Work out the finished part from the listing and answer in its coordinate system (mm). Coordinates: 2 decimals unless noted, no trailing zeros. Order: outer loops, then holes, each group sorted by start corner. A loop starts at its lowest first (then second) coordinate and runs counter-clockwise, first axis right, second up. Notation, with made-up numbers: (18, -34.5) -> (74, -34.5) arc R24 ccw to (74, -20.5) -> close; hole circle Ø7 at (-13, 84). An arc over 180 degrees is marked (long way). Answer as CSV lines item,"result". Start each with the question number.
Item 1: Straight lines are drawn through the part: L1, parallel to Y at x = 740.5, z = 2.5 (3 decimals); L2, parallel to X at y = 1, z = 1.5; L3, parallel to X at y = -0.5, z = -1.5. For each, find the intervals that lie inside material, in ascending order.
Item 2: Section B-B (x = 104.5) is taken. Write down the section's boundary in (y, z) (3 decimals).
Item 3: Section A-A (y = 0) is taken. Write down the section's boundary in (x, z) (3 decimals).
Item 4: This flat-tipped pin is pushed along its axis until it touches: pin 1 Ø4 at (y, z) = (3.5, 0.5) entering from -X. Where does it stop, or does it pass through?
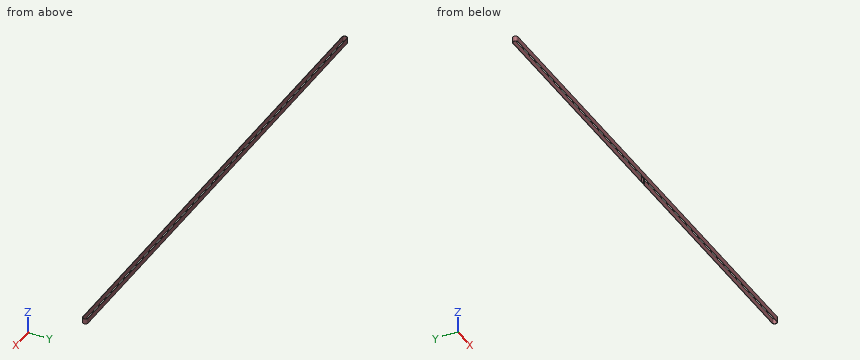
Autodesk Inventor part; units mm, degrees
ref_plane "YZ Plane" through (0, 0, 0) normal (1, 0, 0) x (0, 1, 0)
ref_plane "XZ Plane" through (0, 0, 0) normal (0, 1, 0) x (-1, 0, 0)
ref_plane "XY Plane" through (0, 0, 0) normal (0, 0, 1) x (1, 0, 0)
sketch "_____1" plane through (0, 0, 0) normal (0, 0, 1) x (1, 0, 0)
  arc A0 (0, 4.515) -> (0, -4.515) centre (0, 0) ccw
  line L0 (0, -4.515) -> (837, -4.515)
  arc A1 (837, -4.515) -> (837, 4.515) centre (837, 0) ccw
  line L1 (837, 4.515) -> (0, 4.515)
  arc A2 (0, 3.885) -> (0, -3.885) centre (0, 0) ccw
  line L2 (0, -3.885) -> (837, -3.885)
  arc A3 (837, -3.885) -> (837, 3.885) centre (837, 0) ccw
  line L3 (837, 3.885) -> (0, 3.885)
extrude "Extrusion1" add sketch "_____1" along normal mid plane 9
sketch "_____2" plane through (0, 0, 0) normal (0, 0, 1) x (1, 0, 0)
  line L0 (413.5, 4.515) -> (413.5, 3.885)
  line L1 (413.5, 3.885) -> (413.7598, 3.885)
  arc A0 (413.9085, 3.7546) -> (413.7598, 3.885) centre (413.7598, 3.735) ccw
  arc A1 (413.9085, 3.7546) -> (414.0011, 3.4468) centre (414.9, 3.885) ccw
  arc A2 (414.0011, 3.4468) -> (414.9989, 3.4468) centre (414.5, 3.69) ccw
  arc A3 (414.9989, 3.4468) -> (415.0915, 3.7546) centre (414.1, 3.885) ccw
  arc A4 (415.2402, 3.885) -> (415.0915, 3.7546) centre (415.2402, 3.735) ccw
  line L2 (415.2402, 3.885) -> (415.7598, 3.885)
  arc A5 (415.9085, 3.7546) -> (415.7598, 3.885) centre (415.7598, 3.735) ccw
  arc A6 (415.9085, 3.7546) -> (416.0011, 3.4468) centre (416.9, 3.885) ccw
  arc A7 (416.0011, 3.4468) -> (416.9989, 3.4468) centre (416.5, 3.69) ccw
  arc A8 (416.9989, 3.4468) -> (417.0915, 3.7546) centre (416.1, 3.885) ccw
  arc A9 (417.2402, 3.885) -> (417.0915, 3.7546) centre (417.2402, 3.735) ccw
  line L3 (417.2402, 3.885) -> (417.7598, 3.885)
  arc A10 (417.9085, 3.7546) -> (417.7598, 3.885) centre (417.7598, 3.735) ccw
  arc A11 (417.9085, 3.7546) -> (418.0011, 3.4468) centre (418.9, 3.885) ccw
  arc A12 (418.0011, 3.4468) -> (418.9989, 3.4468) centre (418.5, 3.69) ccw
  arc A13 (418.9989, 3.4468) -> (419.0915, 3.7546) centre (418.1, 3.885) ccw
  arc A14 (419.2402, 3.885) -> (419.0915, 3.7546) centre (419.2402, 3.735) ccw
  line L4 (419.2402, 3.885) -> (419.7598, 3.885)
  arc A15 (419.9085, 3.7546) -> (419.7598, 3.885) centre (419.7598, 3.735) ccw
  arc A16 (419.9085, 3.7546) -> (420.0011, 3.4468) centre (420.9, 3.885) ccw
  arc A17 (420.0011, 3.4468) -> (420.9989, 3.4468) centre (420.5, 3.69) ccw
  arc A18 (420.9989, 3.4468) -> (421.0915, 3.7546) centre (420.1, 3.885) ccw
  arc A19 (421.2402, 3.885) -> (421.0915, 3.7546) centre (421.2402, 3.735) ccw
  line L5 (421.2402, 3.885) -> (421.7598, 3.885)
  arc A20 (421.9085, 3.7546) -> (421.7598, 3.885) centre (421.7598, 3.735) ccw
  arc A21 (421.9085, 3.7546) -> (422.0011, 3.4468) centre (422.9, 3.885) ccw
  arc A22 (422.0011, 3.4468) -> (422.9989, 3.4468) centre (422.5, 3.69) ccw
  arc A23 (422.9989, 3.4468) -> (423.0915, 3.7546) centre (422.1, 3.885) ccw
  arc A24 (423.2402, 3.885) -> (423.0915, 3.7546) centre (423.2402, 3.735) ccw
  line L6 (423.2402, 3.885) -> (423.5, 3.885)
  line L7 (423.5, 3.885) -> (423.5, 4.515)
  line L8 (423.5, 4.515) -> (413.5, 4.515)
extrude "Extrusion2" add sketch "_____2" along normal mid plane 9
properties part number "GBN1700MR2-90_info-1-13-13"
Checked values:
1,L1,"y = -4.515 to -3.885, 3.885 to 4.515"
1,L2,"x = -4.4 to -3.75, 840.75 to 841.4"
1,L3,"x = -4.49 to -3.85, 840.85 to 841.49"
2,outline,"(-4.515, -4.5) -> (-3.885, -4.5) -> (-3.885, 4.5) -> (-4.515, 4.5) -> close; (3.885, -4.5) -> (4.515, -4.5) -> (4.515, 4.5) -> (3.885, 4.5) -> close"
3,outline,"(-4.515, -4.5) -> (-3.885, -4.5) -> (-3.885, 4.5) -> (-4.515, 4.5) -> close; (840.885, -4.5) -> (841.515, -4.5) -> (841.515, 4.5) -> (840.885, 4.5) -> close"
4,pin 1,"stops at x = -4.26"
